```python
from build123d import *

# Parameters (mm, degrees)
ESBO_O2_W                  = 22.9
ESBO_O2_H                  = 12.13
RESSALTO_EXTRUS_O1_DEPTH   = 17.35
ESBO_O3_W                  = 32
ESBO_O3_H                  = 12.13
RESSALTO_EXTRUS_O2_DEPTH   = 2.4
ESBO_O4_W                  = 22.9
ESBO_O4_H                  = 12.13
RESSALTO_EXTRUS_O3_DEPTH   = 4.45
CORTE_EXTRUS_O1_DEPTH      = 2.4
RESSALTO_EXTRUS_O4_DEPTH   = 4.3
ESBO_O7_R                  = 2.45
RESSALTO_EXTRUS_O5_DEPTH   = 3.1
CORTE_EXTRUS_O2_DEPTH      = 1
CORTE_EXTRUS_O2_DEPTH_BACK = 16
ESBO_O10_W                 = 9.190370446
ESBO_O10_H                 = 13.482765879
ESBO_O10_W_2               = 7.294178248
ESBO_O10_H_2               = 14.557386271
RESSALTO_EXTRUS_O7_DEPTH   = 2.4
FILETE1_R                  = 1


with BuildPart() as part:
    # Esboço2 → Ressalto-extrusão1 (new body)
    with BuildSketch(Plane(origin=(0, 0, 0), x_dir=(1, 0, 0), z_dir=(0, 1, 0))):
        Rectangle(ESBO_O2_W, ESBO_O2_H)
    extrude(amount=RESSALTO_EXTRUS_O1_DEPTH)

    # Esboço3 → Ressalto-extrusão2 (add)
    with BuildSketch(Plane(origin=(0, 17.35, 0), x_dir=(1, 0, 0), z_dir=(0, 1, 0))):
        Rectangle(ESBO_O3_W, ESBO_O3_H)
    extrude(amount=RESSALTO_EXTRUS_O2_DEPTH)

    # Esboço4 → Ressalto-extrusão3 (add)
    with BuildSketch(Plane(origin=(0, 19.75, 0), x_dir=(1, 0, 0), z_dir=(0, 1, 0))):
        Rectangle(ESBO_O4_W, ESBO_O4_H)
    extrude(amount=RESSALTO_EXTRUS_O3_DEPTH)

    # Esboço5 → Corte-extrusão1 (cut)
    with BuildSketch(Plane(origin=(0, 19.75, 0), x_dir=(1, 0, 0), z_dir=(0, 1, 0))):
        with BuildLine():
            Line((-16, -0.625), (-16, 0.625))
            Line((-16, 0.625), (-14.707531755, 0.625))
            ThreePointArc((-14.707531755, 0.625), (-12.375, 0), (-14.707531755, -0.625))
            Line((-14.707531755, -0.625), (-16, -0.625))
        make_face()
        with BuildLine():
            Line((14.707531755, -0.625), (16, -0.625))
            Line((16, -0.625), (16, 0.625))
            Line((16, 0.625), (14.707531755, 0.625))
            ThreePointArc((14.707531755, 0.625), (12.375, 0), (14.707531755, -0.625))
        make_face()
    extrude(amount=-CORTE_EXTRUS_O1_DEPTH, mode=Mode.SUBTRACT)

    # Esboço6 → Ressalto-extrusão4 (add)
    with BuildSketch(Plane(origin=(0, 24.2, 0), x_dir=(1, 0, 0), z_dir=(0, 1, 0))):
        with BuildLine():
            Line((-0.55, -2.6), (-0.263142743, -2.6))
            ThreePointArc((-0.263142743, -2.6), (-0.007438587, -2.670331076), (0.176329776, -2.861538462))
            ThreePointArc((0.176329776, -2.861538462), (11.45, 0), (0.176329776, 2.861538462))
            ThreePointArc((0.176329776, 2.861538462), (-0.007438587, 2.670331076), (-0.263142743, 2.6))
            Line((-0.263142743, 2.6), (-0.55, 2.6))
            ThreePointArc((-0.55, 2.6), (-3.15, 0), (-0.55, -2.6))
        make_face()
    extrude(amount=RESSALTO_EXTRUS_O4_DEPTH)

    # Esboço7 → Ressalto-extrusão5 (add)
    with BuildSketch(Plane(origin=(0, 28.5, 0), x_dir=(1, 0, 0), z_dir=(0, 1, 0))):
        with Locations(Location((5.45, 0, 0), (0, 0, 90))):
            Circle(ESBO_O7_R)
    extrude(amount=RESSALTO_EXTRUS_O5_DEPTH)

    # Esboço10 → Corte-extrusão2 (cut, two sides: drawn at the far end of the back side and taken through both)
    with BuildSketch(Plane(origin=(0, 28.5, 0), x_dir=(1, 0, 0), z_dir=(0, 1, 0)).offset(-CORTE_EXTRUS_O2_DEPTH_BACK)):
        with Locations((16.045185223, -0.676382939)):
            Rectangle(ESBO_O10_W, ESBO_O10_H)
        with Locations((-15.097089124, -1.213693136)):
            Rectangle(ESBO_O10_W_2, ESBO_O10_H_2)
    extrude(amount=CORTE_EXTRUS_O2_DEPTH + CORTE_EXTRUS_O2_DEPTH_BACK, mode=Mode.SUBTRACT)

    # Esboço12 → Ressalto-extrusão7 (add)
    with BuildSketch(Plane(origin=(0, 17.6, 0), x_dir=(1, 0, 0), z_dir=(0, 1, 0))):
        with BuildLine():
            Line((16, 0.625), (14.707531755, 0.625))
            ThreePointArc((14.707531755, 0.625), (12.375, 0), (14.707531755, -0.625))
            Line((14.707531755, -0.625), (16, -0.625))
            Line((16, -0.625), (16, -6.065))
            Line((16, -6.065), (11.45, -6.065))
            Line((11.45, -6.065), (11.45, 6.065))
            Line((11.45, 6.065), (16, 6.065))
            Line((16, 6.065), (16, 0.625))
        make_face()
        with BuildLine():
            Line((-16, -0.625), (-16, -6.065))
            Line((-16, -6.065), (-11.45, -6.065))
            Line((-11.45, -6.065), (-11.45, 6.065))
            Line((-11.45, 6.065), (-16, 6.065))
            Line((-16, 6.065), (-16, 0.625))
            Line((-16, 0.625), (-14.707531755, 0.625))
            ThreePointArc((-14.707531755, 0.625), (-12.375, 0), (-14.707531755, -0.625))
            Line((-14.707531755, -0.625), (-16, -0.625))
        make_face()
    extrude(amount=RESSALTO_EXTRUS_O7_DEPTH)

    # Filete1
    filete1_edges = [part.edges().sort_by_distance(p)[0] for p in [
        (11.45, 8.8, 6.065),
        (11.45, 8.8, -6.065),
        (16, 18.8, -6.065),
        (16, 18.8, 6.065),
        (-11.45, 8.8, 6.065),
        (-11.45, 8.8, -6.065),
        (-16, 18.8, 6.065),
        (-16, 18.8, -6.065),
        (-11.45, 22.1, -6.065),
        (11.45, 22.1, -6.065),
        (11.45, 22.1, 6.065),
        (-11.45, 22.1, 6.065),
    ]]
    fillet(filete1_edges, radius=FILETE1_R)


solid = part.part
```
Geometry: final body of the model. Coordinates: model frame, mm. A direction names the side the tool comes from. Give positions to 0.01 mm unless a question says otherwise; leave off trailing zeros. Write each loop counter-clockwise with the first axis right and the second up, starting at its lowest first coordinate (ties: lowest second). Pieces come first, ordered by that corner, then holes.
1. Draft query along Z for faces 5 (the cylindrical face through (11.15, 8.68, -5.78)), 6 (the cylindrical face through (12.376, 18.783, -0.046)), 7 (the cylindrical face through (-12.376, 18.783, -0.046)), 8 (the flat face through (5, 31.6, 0)). Return one class per face: released by +Z, released by -Z, zero draft, split by the parting line, or undercut.
2. Section query C-C, the plane z = -4.25. Return loops of the section in (x, y).
3. Reachability of faces 1 (the cylindrical face through (-3.15, 26.32, -0.06)), 2 (the flat face through (-15, 19, 0.625)), 3 (the cylindrical face through (11.15, 8.68, 5.78)), 4 (the flat face through (11.45, 22, 0)) from +Z, -Z, +X, -X, +Y, -Y: full face, straight path, thin tool, end or side. Return the list, or none.
4. Section query A-A, the plane x = 5.45. Return loops of the section in (y, z) (3 decimals).
5. Pin query (flat end, axial travel): P1, Ø3, axis at x = -13.5, z = 3, coming from the -Y side; P2, Ø3, axis at y = 14.5, z = 4.5, coming from the +X side; P3, Ø4.5, axis at x = 13, z = 0.5, coming from the +Y side. Return the tip coordinate at first contact, or that it passes through.
6. Section query D-D, the plane y = 25.5. Return loops of the section in (x, z), then the cut area to 3 significant figures.
7. Section query B-B, the plane y = 7. Return loops of the section in (x, z) (3 decimals), then the cut area to 3 significant figures.
8. Line query: probe 1 along Y at (x, z) = (-7.5, 0.75); probe 2 along Y at (x, z) = (13, 1.25); probe 3 along X at (y, z) = (8, -2.5). Output: solid intervals per line, ascending.
Computed:
1. face 5: released by -Z
1. face 6: undercut
1. face 7: undercut
1. face 8: zero draft
2. outline: (-16, 17.6) - (-11.45, 17.6) - (-11.45, 0) - (11.45, 0) - (11.45, 17.6) - (16, 17.6) - (16, 20) - (11.45, 20) - (11.45, 24.2) - (9.69, 24.2) - (9.69, 28.5) - (1.21, 28.5) - (1.21, 24.2) - (-11.45, 24.2) - (-11.45, 20) - (-16, 20) - close
3. face 1: -X, +Y
3. face 2: -X, +Y, -Y
3. face 3: +Z, +X, -Y
3. face 4: +Z, -Z, +X, +Y
4. outline: (0, -6.065) - (24.2, -6.065) - (24.2, -6) - (28.5, -6) - (28.5, -2.45) - (31.6, -2.45) - (31.6, 2.45) - (28.5, 2.45) - (28.5, 6) - (24.2, 6) - (24.2, 6.065) - (0, 6.065) - close
5. P1: stops at y = 17.6
5. P2: stops at x = 11.45
5. P3: stops at y = 28.5
6. outline: (-0.55, -2.6) - (-0.26, -2.6) arc R0.5 cw to (0.18, -2.86) arc R6 ccw (long way) to (0.18, 2.86) arc R0.5 cw to (-0.26, 2.6) - (-0.55, 2.6) arc R2.6 ccw to start
6. area: 125 mm2
7. outline: (-11.45, -5.065) arc R1 ccw to (-10.45, -6.065) - (10.45, -6.065) arc R1 ccw to (11.45, -5.065) - (11.45, 5.065) arc R1 ccw to (10.45, 6.065) - (-10.45, 6.065) arc R1 ccw to (-11.45, 5.065) - close
7. area: 277 mm2
8. probe 1: y = 0 to 24.2
8. probe 2: y = 17.6 to 20
8. probe 3: x = -11.45 to 11.45
